Check sheet for the modelled part. Datum: model origin and axes. Units: mm. A direction names the side the tool comes from. Give positions to 0.01 mm unless a question says otherwise; leave off trailing zeros. Write each loop counter-clockwise with the first axis right and the second up, starting at its lowest first coordinate (ties: lowest second). Pieces come first, ordered by that corner, then holes. Notation, with made-up numbers: M 7.25,71.5 L 49.25,71.5 A25 ccw 49.25,84.5 Z; hole C -16.75,51 d8. An arc over 180 degrees is marked long. Write item = value, one per line. Start each with the question number.
1) Access from +Z, -Z, +X, -X, +Y, -Y to the whole of each face (thin tool, end or side, straight path). Record for faces 1 (the flat face through (5, 11, 34)), 2 (the cylindrical face through (24.694, 11.251, 30.071)), 3 (the cylindrical face through (6.752, 11.154, 27.287)).
2) Cross-section at C-C, the plane x = 11.5. Record the cut outline in (y, z), plus the area to 3 significant figures.
3) Scan lines: line 1 along X through (y, z) = (3, 14); line 2 along Y through (x, z) = (19, 29.55); line 3 along Y through (x, z) = (3.5, 15). Record each from-to range of solid material in increasing order. Write a range as [from, to].
4) Mould release check, pull along Y, two halves, no side actions. Record for faces 4 (the cylindrical face through (4.413, 13.763, 6.225)), 5 (the flat face through (32, 8, 21)): released by +Y, released by -Y, zero draft, split by the parting line, or undercut.
5) Cross-section at D-D, the plane z = 4. Record the cut outline in (x, y), plus the area to 3 significant figures.
6) Go/stop test with flat-tipped pins: pin 1 (2 mm diameter, centred on x = 5.5, y = 16.5, fed in from +Z); pin 2 (5.5 mm diameter, centred on y = 8.5, z = 12, fed in from +X). Record where each tip stops, or that it passes through.
7) Cross-section at B-B, the plane z = 30. Record the cut outline in (x, y), plus the area to 3 significant figures.
8) Cross-section at A-A, the plane x = 4. Record the cut outline in (y, z).
```python
from build123d import *

# Parameters (mm, degrees)
SKETCH3_W           = 38
SKETCH3_H           = 34
SKETCH3_W_2         = 26
SKETCH3_H_2         = 22
BOSS_EXTRUDE1_DEPTH = 22
SKETCH4_W           = 24
SKETCH4_H           = 22
BOSS_EXTRUDE2_DEPTH = 1
SKETCH5_R           = 2.7
CUT_EXTRUDE1_DEPTH  = 12
SKETCH7_R           = 5.7
CUT_EXTRUDE3_DEPTH  = 4.2
SKETCH8_R           = 6.2
CUT_EXTRUDE4_DEPTH  = 57.151580565
SKETCH9_R           = 9.2
CUT_EXTRUDE5_DEPTH  = 4.2
SKETCH10_R          = 9.2
CUT_EXTRUDE6_DEPTH  = 4.2
SKETCH15_R          = 1.5
CUT_EXTRUDE7_DEPTH  = 57.151580565
FILLET1_R           = 3
FILLET3_R           = 2.5
FILLET4_R           = 2.2
FILLET5_R           = 2.4


with BuildPart() as part:
    # Sketch3 → Boss-Extrude1 (new body)
    with BuildSketch(Plane(origin=(0, 0, 0), x_dir=(1, 0, 0), z_dir=(0, 1, 0))):
        with Locations((19, -17)):
            Rectangle(SKETCH3_W, SKETCH3_H)
        with Locations((19, -17)):
            Rectangle(SKETCH3_W_2, SKETCH3_H_2, mode=Mode.SUBTRACT)
    extrude(amount=BOSS_EXTRUDE1_DEPTH)

    # Sketch4 → Boss-Extrude2 (add)
    with BuildSketch(Plane.XY.offset(34)):
        with Locations((19, 11)):
            Rectangle(SKETCH4_W, SKETCH4_H)
    extrude(amount=BOSS_EXTRUDE2_DEPTH)

    # Sketch5 → Cut-Extrude1 (cut)
    with BuildSketch(Plane.XY.offset(35)):
        with Locations((19, 11)):
            Circle(SKETCH5_R)
    extrude(amount=-CUT_EXTRUDE1_DEPTH, mode=Mode.SUBTRACT)

    # Sketch7 → Cut-Extrude3 (cut)
    with BuildSketch(Plane(origin=(0, 0, 28), x_dir=(-1, 0, 0), z_dir=(0, 0, -1))):
        with Locations((-19, 11)):
            Circle(SKETCH7_R)
    extrude(amount=-CUT_EXTRUDE3_DEPTH, mode=Mode.SUBTRACT)

    # Sketch8 → Cut-Extrude4 (cut, through all)
    with BuildSketch(Plane(origin=(38, 0, 0), x_dir=(0, 0, -1), z_dir=(1, 0, 0))):
        with Locations((-15, 11)):
            Circle(SKETCH8_R)
    extrude(amount=-CUT_EXTRUDE4_DEPTH, mode=Mode.SUBTRACT)

    # Sketch9 → Cut-Extrude5 (cut)
    with BuildSketch(Plane(origin=(6, 0, 0), x_dir=(0, 0, -1), z_dir=(1, 0, 0))):
        with Locations((-15, 11)):
            Circle(SKETCH9_R)
    extrude(amount=-CUT_EXTRUDE5_DEPTH, mode=Mode.SUBTRACT)

    # Sketch10 → Cut-Extrude6 (cut)
    with BuildSketch(Plane(origin=(38, 0, 0), x_dir=(0, 0, -1), z_dir=(1, 0, 0))):
        with Locations((-15, 11)):
            Circle(SKETCH10_R)
    extrude(amount=-CUT_EXTRUDE6_DEPTH, mode=Mode.SUBTRACT)

    # Sketch15 → Cut-Extrude7 (cut, through all)
    with BuildSketch(Plane(origin=(0, 0, 0), x_dir=(-1, 0, 0), z_dir=(0, -1, 0))):
        with Locations(Location((-4, -30, 0), (0, 0, 90))):
            Circle(SKETCH15_R)
        with Locations(Location((-34, -30, 0), (0, 0, 90))):
            Circle(SKETCH15_R)
        with Locations(Location((-34, -4, 0), (0, 0, 90))):
            Circle(SKETCH15_R)
        with Locations(Location((-4, -4, 0), (0, 0, 90))):
            Circle(SKETCH15_R)
    extrude(amount=-CUT_EXTRUDE7_DEPTH, mode=Mode.SUBTRACT)

    # Fillet1
    # the kernel refuses this fillet: 3 mm, written as the material it takes off along each edge
    with BuildSketch(Plane(origin=(38, -7.5, 0), x_dir=(-1, 0, 0), z_dir=(0, 1, 0)), Plane(origin=(38, -7.5, 34), x_dir=(0, 0, -1), z_dir=(0, 1, 0))) as fillet1_piece_1:
        with BuildLine():
            CenterArc((FILLET1_R, FILLET1_R), FILLET1_R, 180, 90)
            Line((0, FILLET1_R), (-FILLET1_R * 0.02, FILLET1_R))
            Line((-FILLET1_R * 0.02, FILLET1_R), (-FILLET1_R * 0.02, -FILLET1_R * 0.02))
            Line((-FILLET1_R * 0.02, -FILLET1_R * 0.02), (FILLET1_R, -FILLET1_R * 0.02))
            Line((FILLET1_R, -FILLET1_R * 0.02), (FILLET1_R, 0))
        make_face()
    extrude(amount=37, mode=Mode.SUBTRACT)
    with BuildSketch(Plane(origin=(7, -5.590169944, 35), x_dir=(0, 0, -1), z_dir=(0, 1, 0)), Plane(origin=(31, 27.590169944, 35), x_dir=(0, 0, -1), z_dir=(0, -1, 0))) as fillet1_piece_2:
        with BuildLine():
            CenterArc((3, -2.236067977), FILLET1_R, 131.810314896, 48.189685104)
            Line((0, -2.236067977), (-0.06, -2.236067977))
            Line((-0.06, -2.236067977), (-0.06, 0))
            Line((-0.06, 0), (0, 0.06))
            ThreePointArc((0, 0.06), (0.5, 0.06), (0.96, 0.04472136))
            Line((0.96, 0.04472136), (1, 0))
        make_face()
    extrude(amount=33.180339887, mode=Mode.SUBTRACT)
    with BuildSketch(Plane(origin=(0, -7.5, 34), x_dir=(0, 0, -1), z_dir=(0, 1, 0)), Plane(origin=(0, -7.5, 0), x_dir=(1, 0, 0), z_dir=(0, 1, 0))) as fillet1_piece_3:
        with BuildLine():
            CenterArc((FILLET1_R, -FILLET1_R), FILLET1_R, 90, 90)
            Line((0, -FILLET1_R), (-FILLET1_R * 0.02, -FILLET1_R))
            Line((-FILLET1_R * 0.02, -FILLET1_R), (-FILLET1_R * 0.02, FILLET1_R * 0.02))
            Line((-FILLET1_R * 0.02, FILLET1_R * 0.02), (FILLET1_R, FILLET1_R * 0.02))
            Line((FILLET1_R, FILLET1_R * 0.02), (FILLET1_R, 0))
        make_face()
    extrude(amount=37, mode=Mode.SUBTRACT)

    # Fillet3
    fillet3_edges = [part.edges().sort_by_distance(p)[0] for p in [
        (6, 11, 28),
        (32, 11, 6),
    ]]
    fillet(fillet3_edges, radius=FILLET3_R)

    # Fillet4
    fillet4_edges = [part.edges().sort_by_distance(p)[0] for p in [
        (32, 11, 28),
    ]]
    fillet(fillet4_edges, radius=FILLET4_R)

    # Fillet5
    # the kernel refuses this fillet: 2.4 mm, written as the material it adds along each edge
    with BuildSketch(Plane(origin=(6, 6.907878403, 6), x_dir=(0, 0, 1), z_dir=(0, 1, 0))) as fillet5_piece_1_section:
        with BuildLine():
            CenterArc((FILLET5_R, FILLET5_R), FILLET5_R, 180, 90)
            Line((0, FILLET5_R), (0, 0))
            Line((0, 0), (FILLET5_R, 0))
        make_face()
    fillet5_piece_1 = extrude(amount=15.092121597, mode=Mode.PRIVATE)
    fillet5_piece_1 = fillet5_piece_1 - Plane(origin=(6.778295216, 11, 15), x_dir=(0, 0, -1), z_dir=(1, 0, 0)) * Cylinder(9.2, 40, mode=Mode.PRIVATE)
    add(fillet5_piece_1)
    with BuildSketch(Plane(origin=(6, 0, 6), x_dir=(0, 0, 1), z_dir=(0, 1, 0))) as fillet5_piece_2_section:
        with BuildLine():
            CenterArc((FILLET5_R, FILLET5_R), FILLET5_R, 180, 90)
            Line((0, FILLET5_R), (0, 0))
            Line((0, 0), (FILLET5_R, 0))
        make_face()
    fillet5_piece_2 = extrude(amount=15.092121597, mode=Mode.PRIVATE)
    fillet5_piece_2 = fillet5_piece_2 - Plane(origin=(6.572967992, 11, 15), x_dir=(0, 0, -1), z_dir=(1, 0, 0)) * Cylinder(9.2, 40, mode=Mode.PRIVATE)
    add(fillet5_piece_2)


solid = part.part
```
Reply:
q1.face_1 = +Z, -X, +Y, -Y
q1.face_2 = none
q1.face_3 = +Y, -Y
q2.outline = M 0,0 L 22,0 L 22,6 L 0,6 Z; M 0,28 L 22,28 L 22,35 L 0,35 Z
q2.area = 286 mm2
q3.line_1 = [0, 1.8], [32, 33.8]
q3.line_2 = [0, 5.3], [16.7, 22]
q3.line_3 = [0, 1.8], [20.2, 22]
q4.face_4 = undercut
q4.face_5 = zero draft
q5.outline = M 0,0 L 2.5,0 L 2.5,22 L 0,22 Z; M 5.5,0 L 32.5,0 L 32.5,22 L 5.5,22 Z; M 35.5,0 L 38,0 L 38,22 L 35.5,22 Z
q5.area = 704 mm2
q6.pin_1 = 34
q6.pin_2 = 33.8
q7.outline = M 0,0 L 2.5,0 L 2.5,22 L 0,22 Z; M 5.5,0 L 32.5,0 L 32.5,22 L 5.5,22 Z; M 35.5,0 L 38,0 L 38,22 L 35.5,22 Z; hole C 19,11 d11.4
q7.area = 602 mm2
q8.outline = M 0,0 L 22,0 L 22,2.5 L 0,2.5 Z; M 0,5.5 L 22,5.5 L 22,28.5 L 0,28.5 Z; M 0,31.5 L 22,31.5 L 22,34 L 0,34 Z; hole C 11,15 d18.4
